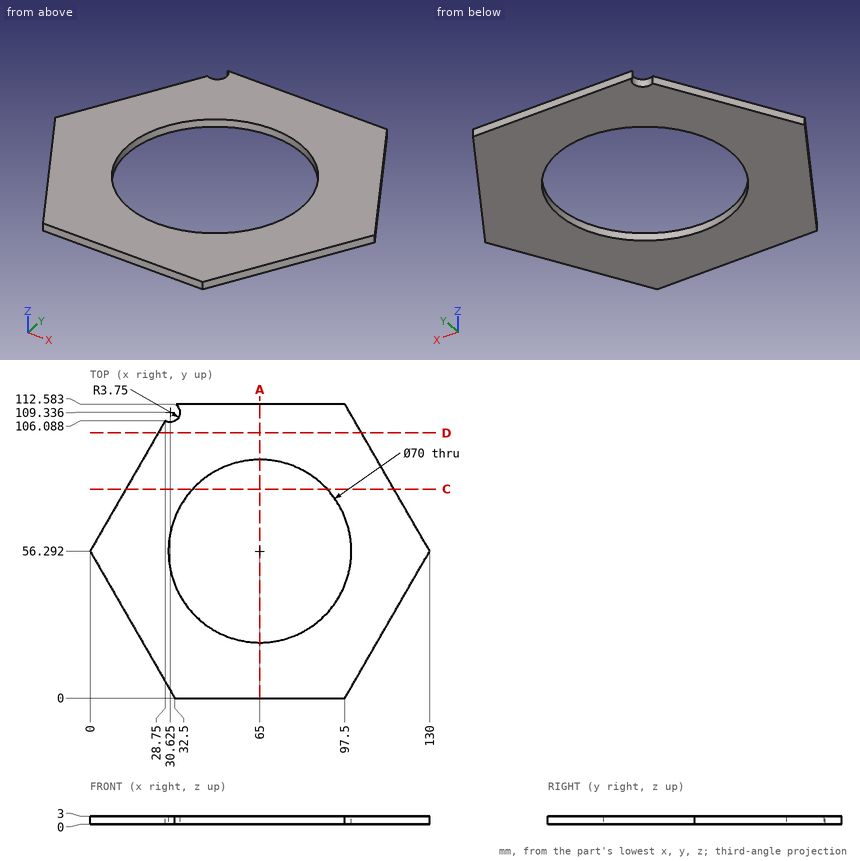
Check sheet for the drawn part. Datum: minimum x, y, z corner. Units: mm. Round coordinates to 2 decimals unless told otherwise and drop trailing zeros. Loops run counter-clockwise (first coordinate to the right, second up) from the corner with the lowest first, then second, coordinate; pieces in that order, holes last. Notation, with made-up numbers: (83.25, -2.5) -> (115.25, -2.5) arc R22 ccw to (115.25, 5.5) -> close; hole circle Ø1 at (-27.75, -23). An arc over 180 degrees is marked (long way). Put each result on its own line as item: value. Start each with the question number.
1. Section check A-A (x = 65). Enter the section's corners in (y, z), plus the area to 3 significant figures.
2. Scan lines: probe 1 along Y at (x, z) = (65, 0.95); probe 2 along X at (y, z) = (62, 1.25) (1 decimal); probe 3 along X at (y, z) = (84.5, 1.55) (1 decimal). Record each from-to range of solid material in increasing order.
3. Section check C-C (y = 80). Enter the section's corners in (x, z), plus the area to 3 significant figures.
4. Section check D-D (y = 101.5). Enter the section's corners in (x, z).
Findings:
1. outline: (0, 0) -> (21.29, 0) -> (21.29, 3) -> (0, 3) -> close; (91.29, 0) -> (112.58, 0) -> (112.58, 3) -> (91.29, 3) -> close
1. area: 128 mm^2
2. probe 1: y = 0 to 21.29, 91.29 to 112.58
2. probe 2: x = 3.3 to 30.5, 99.5 to 126.7
2. probe 3: x = 16.3 to 44.3, 85.7 to 113.7
3. outline: (13.69, 0) -> (39.25, 0) -> (39.25, 3) -> (13.69, 3) -> close; (90.75, 0) -> (116.31, 0) -> (116.31, 3) -> (90.75, 3) -> close
3. area: 153 mm^2
4. outline: (26.1, 0) -> (103.9, 0) -> (103.9, 3) -> (26.1, 3) -> close
